Geometry: final body of the model. Coordinates: model frame, mm. A direction names the side the tool comes from. Give positions to 0.01 mm unless a question says otherwise; leave off trailing zeros. Write each loop counter-clockwise with the first axis right and the second up, starting at its lowest first coordinate (ties: lowest second). Pieces come first, ordered by that corner, then holes. Notation, with made-up numbers: (-29, 62.25) -> (-18, 62.25) arc R26 cw to (-18, 89.25) -> close; hole circle Ø4 at (-38, -34). An arc over 180 degrees is marked (long way). Answer as a JSON object with one key per item and string values. Group by question number.
(1) Section query C-C on z = -12.7. State how many separate pieces and enclosed holes the cut face has, plus the area to 3 significant figures.
(2) Material intervals for probe 1 along X at (y, z) = (1.25, -12.7); probe 2 along Z at (x, y) = (-12.7, 2.05); probe 3 along Y at (x, z) = (-35.5, -19.75), sorted ascending.
(3) Set-up query: faces 5 (the face through (-276.226, 1.69, -13.405)), 6 (the face through (-154, 10, -21.793)). Return all of +Z, -Z, +X, -X, +Y, -Y with unobstructed straight access to the full face (end or side cutting, diameter ignored); none if empty.
(4) Section query B-B on y = 8.5. Output: boundary loops of the cut face in (x, z), plus the area to 3 significant figures.
(5) Section query D-D on x = -122. Output: boundary loops of the cut face in (y, z).
(6) Contact query for flat-ended pins moving along their axis: pin 1 Ø3 at (x, y) = (-62, 10.5) entering from +Z; pin 2 Ø1.1 at (y, z) = (12, -23) entering from +X; pin 3 Ø4 at (x, z) = (-279.4, -12.7) entering from -Y; pin 4 Ø1.1 at (y, z) = (9.5, -24) entering from -X. Output: stop coordinate, or through.
(7) Draft query along Z for faces 1 (the face through (-371.524, 1.69, -13.123)), 2 (the face through (-318, 10, -21.793)), 3 (the face through (-193, 19.456, -13)), 4 (the face through (-15.924, 17.718, -13.123)). Return one class per face: +Z half, -Z half, draft (parallel to the pull), parting line (faces both ways), or undercut.
(8) Section query A-A on x = -279.4. Output: boundary loops of the cut face in (y, z), plus the area to 3 significant figures.
Autodesk Inventor part; units mm, degrees
ref_plane "YZ Plane" through (0, 0, 0) normal (1, 0, 0) x (0, 1, 0)
ref_plane "XZ Plane" through (0, 0, 0) normal (0, 1, 0) x (-1, 0, 0)
ref_plane "XY Plane" through (0, 0, 0) normal (0, 0, 1) x (1, 0, 0)
sketch "Sketch1" plane through (0, 0, 0) normal (0, 1, 0) x (-1, 0, 0)
  line L0 (0, 0) -> (381, 0)
  line L1 (381, 0) -> (381, -25.4)
  line L2 (381, -25.4) -> (0, -25.4)
  line L3 (0, -25.4) -> (0, 0)
  dimension "d0" = 381
  dimension "d1" = 25.4
extrude "Extrusion1" add sketch "Sketch1" along normal blind 3.429
sketch "Sketch2" plane through (0, 3.429, 0) normal (0, 1, 0) x (1, 0, 0)
  line L0 (0, 25.4) -> (-381, 25.4)
  line L1 (-38.1, 25.4) -> (-266.7, 25.4)
  line L2 (-266.7, 25.4) -> (-266.7, 21.7932)
  line L3 (-266.7, 21.7932) -> (-38.1, 21.7932)
  line L4 (-38.1, 21.7932) -> (-38.1, 25.4)
  line L5 (0, 0) -> (0, 25.4)
  line L6 (-292.1, 25.4) -> (-342.9, 25.4)
  line L7 (-342.9, 25.4) -> (-342.9, 21.7932)
  line L8 (-342.9, 21.7932) -> (-292.1, 21.7932)
  line L9 (-292.1, 21.7932) -> (-292.1, 25.4)
  point P0 (-266.7, 23.5966)
  dimension "d4" = 228.6
  dimension "d5" = 3.6068
  dimension "d6" = 38.1
  dimension "d7" = 50.8
  dimension "d8" = 3.6068
  dimension "d9" = 25.4
extrude "Extrusion2" add sketch "Sketch2" along normal blind 12.5984
sketch "Sketch3" plane through (0, 16.0274, 0) normal (0, 1, 0) x (1, 0, 0)
  line L0 (-381, 0) -> (0, 0)
  line L1 (0, 25.4) -> (-381, 25.4)
  line L2 (-381, 0) -> (0, 0)
  line L3 (0, 0) -> (0, 25.4)
  line L4 (0, 25.4) -> (-381, 25.4)
  line L5 (-381, 25.4) -> (-381, 0)
extrude "Extrusion3" add sketch "Sketch3" along normal blind 3.429
sketch "Sketch4" plane through (0, 19.4564, 0) normal (0, 1, 0) x (1, 0, 0)
  line L0 (0, 25.4) -> (-381, 25.4)
  line L1 (0, 0) -> (0, 25.4)
  point P0 (-12.7, 12.7)
  dimension "d14" = 12.7
  dimension "d15" = 12.7
hole "Hole1" at (-12.7, 19.4564, -12.7) direction (0, -1, 0) diameter 6.5024 end through all
sketch "Sketch5" plane through (0, 19.4564, 0) normal (0, 1, 0) x (1, 0, 0)
  line L0 (0, 25.4) -> (-381, 25.4)
  line L1 (-381, 25.4) -> (-381, 0)
  point P0 (0, 0)
  point P1 (-279.4, 12.7)
  point P2 (-381, 12.7)
  dimension "d23" = 12.7
  dimension "d40" = 101.6
hole "Hole2" at (-279.4, 19.4564, -12.7) direction (0, -1, 0) diameter 6.5024 end through all
sketch "Sketch6" plane through (0, 19.4564, 0) normal (0, 1, 0) x (1, 0, 0)
  line L0 (0, 25.4) -> (-381, 25.4)
  line L1 (-381, 25.4) -> (-381, 0)
  point P0 (0, 0)
  point P1 (-368.3, 12.7)
  dimension "d31" = 12.7
  dimension "d32" = 12.7
hole "Hole3" at (-368.3, 19.4564, -12.7) direction (0, -1, 0) diameter 6.5024 end through all
properties part number "ArmPart3"
Answer list:
{
 "1": {"separate pieces": "8", "enclosed holes": "0", "area": "2,480 mm2"},
 "2": {"probe 1": "-381 to -371.55, -365.05 to -282.65, -276.15 to -15.95, -9.45 to 0", "probe 2": "-25.4 to -15.95, -9.45 to 0", "probe 3": "0 to 3.43, 16.03 to 19.46"},
 "3": {"face 5": "+Y, -Y", "face 6": "+Z, +X, -X"},
 "4": {"outline": "(-342.9, -25.4) -> (-292.1, -25.4) -> (-292.1, -21.79) -> (-342.9, -21.79) -> close; (-266.7, -25.4) -> (-38.1, -25.4) -> (-38.1, -21.79) -> (-266.7, -21.79) -> close", "area": "1,010 mm2"},
 "5": {"outline": "(0, -25.4) -> (19.46, -25.4) -> (19.46, 0) -> (16.03, 0) -> (16.03, -21.79) -> (3.43, -21.79) -> (3.43, 0) -> (0, 0) -> close"},
 "6": {"pin 1": "z = -21.79", "pin 2": "x = -38.1", "pin 3": "through", "pin 4": "x = -342.9"},
 "7": {"face 1": "undercut", "face 2": "+Z half", "face 3": "draft", "face 4": "undercut"},
 "8": {"outline": "(0, -25.4) -> (3.43, -25.4) -> (3.43, -15.95) -> (0, -15.95) -> close; (0, -9.45) -> (3.43, -9.45) -> (3.43, 0) -> (0, 0) -> close; (16.03, -25.4) -> (19.46, -25.4) -> (19.46, -15.95) -> (16.03, -15.95) -> close; (16.03, -9.45) -> (19.46, -9.45) -> (19.46, 0) -> (16.03, 0) -> close", "area": "130 mm2"}
}
